Part print with two shaded views. Sizes in mm from the minimum x, y, z corner. A direction names the side the tool comes from. Give positions to 0.01 mm unless a question says otherwise; leave off trailing zeros. Order: outer loops, then holes, each group sorted by start corner. A loop starts at its lowest first (then second) coordinate and runs counter-clockwise, first axis right, second up. Notation, with made-up numbers: (39.25, -10) -> (54.25, -10) arc R25 cw to (54.25, 2) -> close; hole circle Ø8 at (-27, 10). An arc over 180 degrees is marked (long way). Write item = value, one per line. Start each with the question number.
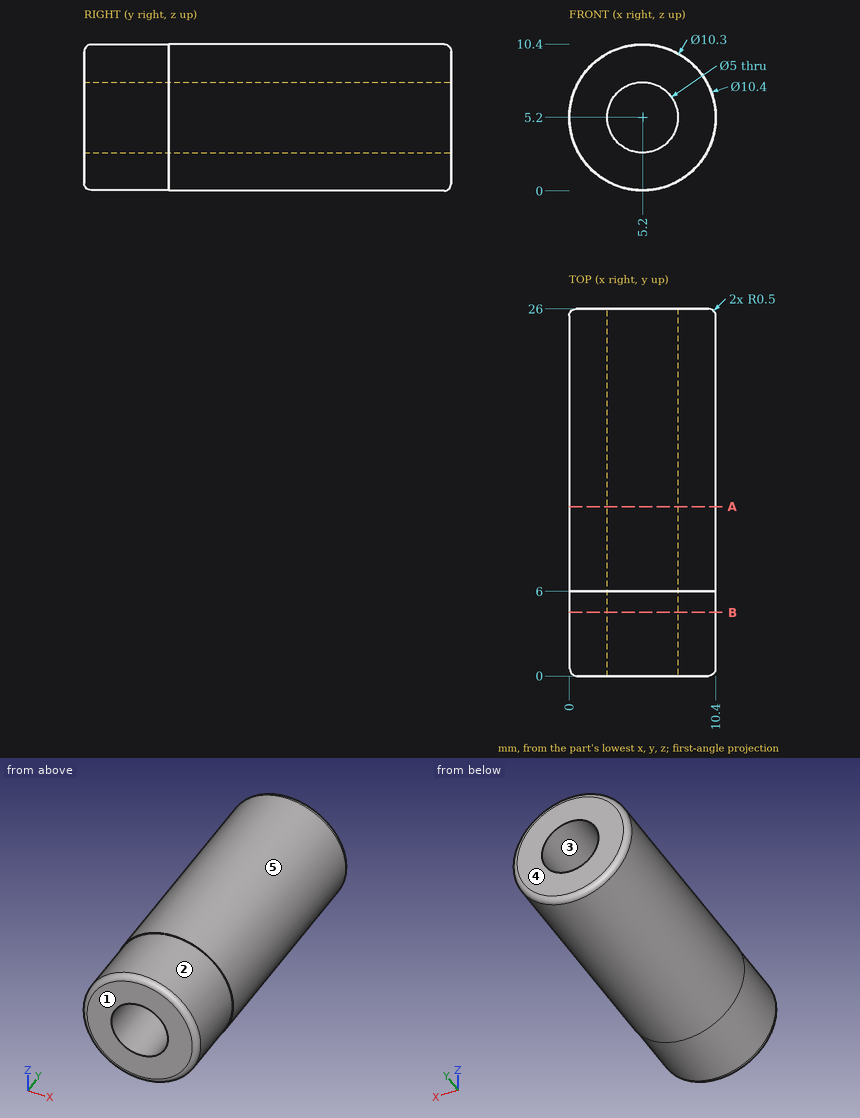
(1) Cut at B-B, the plane y = 4.5. Give the cut face in (x, z), plus the area to 3 significant figures.
(2) 3-axis set-ups, long thin cutter, end or side, ignore diameter. For the marked faces 1 and 2: which of +Z, -Z, +X, -X, +Y, -Y reach the whole face in a straight line?
(3) Flat gauge pins, fed straight in: P1, Ø1.5, axis at x = 6.5, y = 12.5, coming from the -Z side; P2, Ø2, axis at y = 9, z = 7.5, coming from the -X side. Where does each tip first touch, or does it go through?
(4) Wall check: line 1 (Z direction, x = 5.2, y = 17.75); line 2 (X direction, y = 18, z = 7.25); line 3 (Z direction, x = 5.75, y = 12.5). Give the ranges that are in metal, low to high. Write a range as [from, to].
(5) Mould opens along X. For the marked faces 3, 4 and 5 say: released by +X, released by -X, zero draft, split by the parting line, or undercut.
(6) Cut at A-A, the plane y = 12. Give the cut face in (x, z).
Results:
q1.outline = circle Ø10.3 at (5.2, 5.2); hole circle Ø5 at (5.2, 5.2)
q1.area = 63.7 mm2
q2.face_1 = +Z, -Z, +X, -X, -Y
q2.face_2 = -Y
q3.P1 = 0.03
q3.P2 = 0.17
q4.line_1 = [0, 2.7], [7.7, 10.4]
q4.line_2 = [0.42, 3.77], [6.63, 9.98]
q4.line_3 = [0.03, 2.76], [7.64, 10.37]
q5.face_3 = undercut
q5.face_4 = zero draft
q5.face_5 = split by the parting line
q6.outline = circle Ø10.4 at (5.2, 5.2); hole circle Ø5 at (5.2, 5.2)
